```python
from build123d import *

# Parameters (mm, degrees)
F0_R     = 25
F1_DEPTH = 8
F2_R     = 20
F3_DEPTH = 10
F4_R     = 19
F5_DEPTH = 5
F6_R     = 20
F7_DEPTH = 10
F8_R     = 17.5
F9_DEPTH = 25


with BuildPart() as f1:
    # F0 (on Top) → F1 (new body)
    with BuildSketch(Plane.XY):
        Circle(F0_R)
    extrude(amount=F1_DEPTH)



with BuildPart() as f3:
    # F2 (on face) → F3 (new body)
    with BuildSketch(Plane.XY.offset(23)):
        Circle(F2_R)
    extrude(amount=F3_DEPTH)

    # F4 (on face) → F5 (join)
    with BuildSketch(Plane.XY.offset(18)):
        Circle(F4_R)
    extrude(amount=F5_DEPTH)


with BuildPart() as f1_1:
    add(f1.part)

    add(f3.part)  # F7 merges F3
    # F6 (on face) → F7 (join)
    with BuildSketch(Plane.XY.offset(8)):
        Circle(F6_R)
    extrude(amount=F7_DEPTH)

    # F8 (on face) → F9 (cut)
    with BuildSketch(Plane(origin=(0, 0, 0), x_dir=(1, 0, 0), z_dir=(0, 0, -1))):
        Circle(F8_R)
    extrude(amount=-F9_DEPTH, mode=Mode.SUBTRACT)


solid = f1_1.part
```
Verification items for the finished model (mm, model axes). A direction names the side the tool comes from. Coordinates: 2 decimals unless noted, no trailing zeros. Order: outer loops, then holes, each group sorted by start corner. A loop starts at its lowest first (then second) coordinate and runs counter-clockwise, first axis right, second up. Notation, with made-up numbers: (-6.75, 12.25) -> (37.25, 12.25) arc R15 ccw to (37.25, 35.25) -> close; hole circle Ø1 at (20.5, -37.75). An arc over 180 degrees is marked (long way). Answer as CSV lines item,"result". Start each with the question number.
1) Gauge pin test, flat ends, axial feed: pin 1 Ø10 at (y, z) = (-15.5, 6.5) entering from -X; pin 2 Ø4 at (y, z) = (-19, 25.5) entering from +X; pin 3 Ø1.5 at (y, z) = (9, 19.5) entering from -X. Record the tip position at first contact, or that the pin passes through.
2) Cross-section at A-A, the plane y = 0. Record the boundary of the cut face in (x, z).
3) Cross-section at D-D, the plane z = 7. Record the boundary of the cut face in (x, y).
4) Material ranges on L1, parallel to Y at x = 0, z = 15.75; L2, parallel to Y at x = 0, z = 5.5; L3, parallel to Z at x = -5.5, y = 18.5, recorded low to high. Write a range as [from, to].
5) Set-up check for faces 4 (the face through (18, -7, 23)), 5 (the face through (0, 0, 25)), 6 (the face through (-11, 17, 8)): record each of +Z, -Z, +X, -X, +Y, -Y from which the full face is reachable in a straight line by a thin tool's end or side.
6) Cross-section at C-C, the plane z = 15.5. Record the boundary of the cut face in (x, y).
7) Release check for a two-part mould opening along Y. For faces 1 (the face through (-13.887, 10.648, 12.325)), 2 (the face through (8.767, -16.856, 20.465)), 3 (the face through (18, -7, 18)) record: released by +Y, released by -Y, zero draft, split by the parting line, or undercut.
Conclusion:
1,pin 1,"stops at x = -22.69"
1,pin 2,"stops at x = 10.54"
1,pin 3,"stops at x = -17.12"
2,outline,"(-25, 0) -> (-17.5, 0) -> (-17.5, 25) -> (17.5, 25) -> (17.5, 0) -> (25, 0) -> (25, 8) -> (20, 8) -> (20, 18) -> (19, 18) -> (19, 23) -> (20, 23) -> (20, 33) -> (-20, 33) -> (-20, 23) -> (-19, 23) -> (-19, 18) -> (-20, 18) -> (-20, 8) -> (-25, 8) -> close"
3,outline,"circle Ø50 at (0, 0); hole circle Ø35 at (0, 0)"
4,L1,"y = [-20, -17.5], [17.5, 20]"
4,L2,"y = [-25, -17.5], [17.5, 25]"
4,L3,"z = [0, 18], [23, 33]"
5,face 4,"none"
5,face 5,"-Z"
5,face 6,"+Z"
6,outline,"circle Ø40 at (0, 0); hole circle Ø35 at (0, 0)"
7,face 1,"undercut"
7,face 2,"split by the parting line"
7,face 3,"zero draft"
